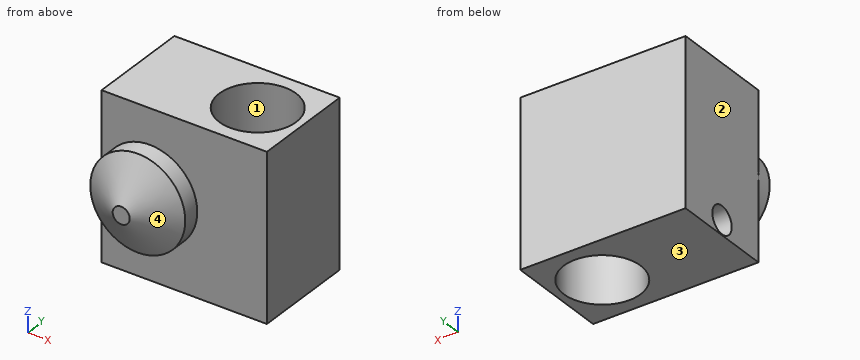
```python
from build123d import *

# Parameters (mm, degrees)
SKETCH1_W           = 12.7
SKETCH1_H           = 12.7
BOSS_EXTRUDE1_DEPTH = 7.9
SKETCH2_R           = 2.95
CUT_EXTRUDE1_DEPTH  = 17.248769184
SKETCH3_R           = 3.65
BOSS_EXTRUDE2_DEPTH = 3.1
CHAMFER1_SIZE       = 1.8
CHAMFER1_SIZE2      = 2.995703068
SKETCH4_R           = 1.05
CUT_EXTRUDE2_DEPTH  = 4


with BuildPart() as part:
    # Sketch1 → Boss-Extrude1 (new body)
    with BuildSketch(Plane(origin=(0, 0, 0), x_dir=(1, 0, 0), z_dir=(0, 1, 0))):
        Rectangle(SKETCH1_W, SKETCH1_H)
    extrude(amount=BOSS_EXTRUDE1_DEPTH)

    # Sketch2 → Cut-Extrude1 (cut, through all)
    with BuildSketch(Plane.XY.offset(6.35)):
        with Locations((2.85, 3.95)):
            Circle(SKETCH2_R)
    extrude(amount=-CUT_EXTRUDE1_DEPTH, mode=Mode.SUBTRACT)

    # Sketch3 → Boss-Extrude2 (add)
    with BuildSketch(Plane.XZ):
        with Locations(Location((-2.65, 0, 0), (0, 0, 270))):
            Circle(SKETCH3_R)
    extrude(amount=BOSS_EXTRUDE2_DEPTH)

    # Chamfer1
    chamfer1_edges = [part.edges().sort_by_distance(p)[0] for p in [
        (-2.65, -3.1, 3.65),
    ]]
    chamfer1_side = [part.faces().sort_by_distance(p)[0] for p in [
        (-2.65, -1.55, 3.65),
    ]]
    chamfer(chamfer1_edges, length=CHAMFER1_SIZE, length2=CHAMFER1_SIZE2, reference=chamfer1_side[0])

    # Sketch4 → Cut-Extrude2 (cut)
    with BuildSketch(Plane.ZY.offset(6.35)):
        with Locations((-5.225, 3.95)):
            Circle(SKETCH4_R)
    extrude(amount=-CUT_EXTRUDE2_DEPTH, mode=Mode.SUBTRACT)


solid = part.part
```
Could you check a few things on this model? Use its own coordinates, in mm. Face numbers are marked on the shaded views. Give positions to 0.01 mm unless a question says otherwise; leave off trailing zeros. Loops run counter-clockwise (first coordinate to the right, second up) from the corner with the lowest first, then second, coordinate; pieces in that order, holes last. Notation, with made-up numbers: (30.25, 52.25) - (67.25, 52.25) arc R17 cw to (67.25, 80.25) - close; hole circle Ø8 at (-13, 1.25). An arc over 180 degrees is marked (long way). Use one line per item in the form item = value.
1. I want a section at D-D (z = 0). Please give me the cut outline in (x, y), and give its area (3 significant figures).
Response values:
outline = (-6.35, 0) - (-6.3, 0) - (-6.3, -1.3) - (-3.3, -3.1) - (-2, -3.1) - (1, -1.3) - (1, 0) - (6.35, 0) - (6.35, 7.9) - (-6.35, 7.9) - close; hole circle Ø5.9 at (2.85, 3.95)
area = 90.2 mm²
2. I need wall thicknesses on probe 1 along Y at (x, z) = (2.85, 2); probe 2 along X at (y, z) = (4.75, 0.5); probe 3 along Y at (x, z) = (-1, 3.75). Which ranges of each line are inside material? Lowest first, please.
Response values:
probe_1 = 0 to 1, 6.9 to 7.9
probe_2 = -6.35 to 0.01, 5.69 to 6.35
probe_3 = 0 to 7.9
3. Thinking about a two-plate mould opening in X: for the marked faces 1, 2, 3 and 4, which applies, released by +X, released by -X, zero draft, split by the parting line, or undercut?
Response values:
face_1 = undercut
face_2 = released by -X
face_3 = zero draft
face_4 = split by the parting line
4. I want a section at B-B (y = 3.95). Please give me the cut outline in (x, z) (3 decimals), and give its area (3 significant figures).
Response values:
outline = (-6.35, -6.35) - (-0.1, -6.35) - (-0.1, 6.35) - (-6.35, 6.35) - (-6.35, -4.175) - (-2.35, -4.175) - (-2.35, -6.275) - (-6.35, -6.275) - close; (5.8, -6.35) - (6.35, -6.35) - (6.35, 6.35) - (5.8, 6.35) - close
area = 78.0 mm²
5. I want a section at A-A (x = 2.85). Please give me the cut outline in (y, z).
Response values:
outline = (0, -6.35) - (1, -6.35) - (1, 6.35) - (0, 6.35) - close; (6.9, -6.35) - (7.9, -6.35) - (7.9, 6.35) - (6.9, 6.35) - close
6. I want a section at C-C (z = 4.75). Please give me the cut outline in (x, y).
Response values:
outline = (-6.35, 0) - (6.35, 0) - (6.35, 7.9) - (-6.35, 7.9) - close; hole circle Ø5.9 at (2.85, 3.95)
